```python
from build123d import *

# Parameters (mm, degrees)
F2_R     = 146.304
F3_DEPTH = 12.7


with BuildPart() as f1:
    # F0 (on Front) → F1 (revolve)
    with BuildSketch(Plane.XZ):
        Polygon((0, 155.829), (0, 152.4), (25.4, 142.875), (25.4, 146.304), align=None)
    revolve(axis=Axis((14.760356, 0, 0), (1, 0, 0)))

    # F2 (on face) → F3 (join)
    with BuildSketch(Plane.YZ.offset(25.4)):
        Circle(F2_R)
    extrude(amount=F3_DEPTH)

    # F4 (on Front) → F5 (revolve, cut)
    with BuildSketch(Plane.XZ):
        Polygon((31.113731, 125.831813), (25.4, 125.831813), (25.4, 0), (38.1, 0), (38.1, 119.858369), (31.113731, 119.858369), align=None)
    revolve(axis=Axis((39.318715, 0, 0), (1, 0, 0)), mode=Mode.SUBTRACT)


solid = f1.part
```
For this review, take the finished solid that the model builds, in its own axes (mm). A direction names the side the tool comes from. Round coordinates to 2 decimals unless told otherwise and drop trailing zeros. Order: outer loops, then holes, each group sorted by start corner. A loop starts at its lowest first (then second) coordinate and runs counter-clockwise, first axis right, second up.
Q1. We need section C-C, the plane x = 14. Give the boundary of the cut face in (y, z).
Findings below:
outline: circle Ø301.16 at (0, 0); hole circle Ø294.3 at (0, 0)
Q2. Insertion check: P1, Ø1.5, axis at x = 5.5, y = -13, coming from the -Z side; P2, Ø5, axis at x = 19.5, z = -84, coming from the +Y side; P3, Ø3, axis at x = 17.5, y = -90, coming from the +Z side. Each pin has a flat end and moves straight along its axis. Give the tip position at first contact, or say it passes through.
Findings below:
P1: stops at z = -153.51
P2: stops at y = 124.5
P3: stops at z = 120.4
Q3. Mouldability with a two-part tool opening along Z and no side actions: class faces 3 (the cylindrical face through (31.661, -31.716, -142.825)), 4 (the flat face through (0, 149, 34)), 5 (the cylindrical face through (28.22, -37.8, 120.02)) as pulls with the +Z half, pulls with the -Z half, needs draft (parallel to the pull), parting line crosses it, or undercut.
Findings below:
face 3: parting line crosses it
face 4: needs draft
face 5: undercut
Q4. Wall thickness on line 1 (Y direction, x = 35.5, z = 0); line 2 (Y direction, x = 29.3, z = 0): over which ranges is each line inside the solid? List them lowest first.
Findings below:
line 1: y = -146.3 to -119.86, 119.86 to 146.3
line 2: y = -146.3 to -125.83, 125.83 to 146.3
Q5. We need section A-A, the plane z = 0. Give the boundary of the cut face in (x, y) (3 decimals).
Findings below:
outline: (0, -155.829) - (25.4, -146.304) - (38.1, -146.304) - (38.1, -119.858) - (31.114, -119.858) - (31.114, -125.832) - (25.4, -125.832) - (25.4, -142.875) - (0, -152.4) - close; (0, 152.4) - (25.4, 142.875) - (25.4, 125.832) - (31.114, 125.832) - (31.114, 119.858) - (38.1, 119.858) - (38.1, 146.304) - (25.4, 146.304) - (0, 155.829) - close
Q6. Machinability: for faces 1 (the flat face through (25.4, -1, -126)), 2 (the flat face through (38.1, -55, -108)), which of the approach directions +Z, -Z, +X, -X, +Y, -Y give a long, thin tool a straight path to every point of the face, cutting with its end or side? Answer none if there is none.
Findings below:
face 1: -X
face 2: +Z, -Z, +X, +Y, -Y
